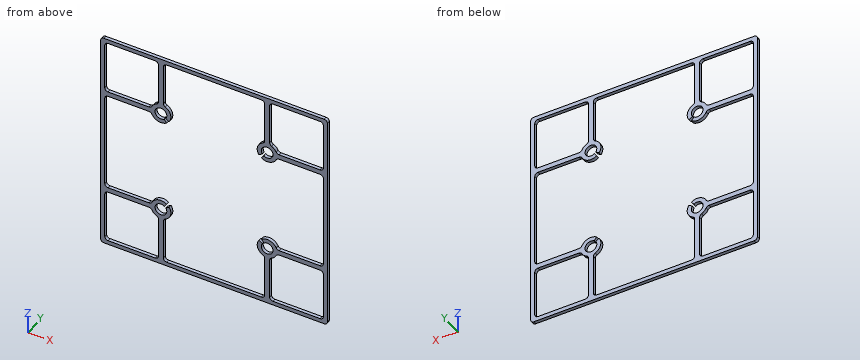
from build123d import *

# Parameters (mm, degrees)
BOSS_EXTRUDE2_DEPTH = 2


with BuildPart() as part:
    # Sketch1 → Boss-Extrude2 (new body)
    with BuildSketch(Plane(origin=(0, 0, 0), x_dir=(1, 0, 0), z_dir=(0, 1, 0))):
        with BuildLine():
            Line((69.363368179, -67.363368179), (69.363368179, 67.363368179))
            ThreePointArc((69.363368179, 67.363368179), (68.777581741, 68.777581741), (67.363368179, 69.363368179))
            Line((67.363368179, 69.363368179), (-67.363368179, 69.363368179))
            ThreePointArc((-67.363368179, 69.363368179), (-68.777581741, 68.777581741), (-69.363368179, 67.363368179))
            Line((-69.363368179, 67.363368179), (-69.363368179, -67.363368179))
            ThreePointArc((-69.363368179, -67.363368179), (-68.777581741, -68.777581741), (-67.363368179, -69.363368179))
            Line((-67.363368179, -69.363368179), (67.363368179, -69.363368179))
            ThreePointArc((67.363368179, -69.363368179), (68.777581741, -68.777581741), (69.363368179, -67.363368179))
        make_face()
        with BuildLine():
            Line((66.863368179, -64.863368179), (66.863368179, -35.99568434))
            ThreePointArc((66.863368179, -35.99568434), (66.277581741, -34.581470778), (64.863368179, -33.99568434))
            Line((64.863368179, -33.99568434), (39.806859174, -33.99568434))
            ThreePointArc((39.806859174, -33.99568434), (38.740619021, -34.303605165), (38.002696415, -35.132552404))
            ThreePointArc((38.002696415, -35.132552404), (36.814625157, -36.812077197), (35.135802469, -38.001140368))
            ThreePointArc((35.135802469, -38.001140368), (34.307605976, -38.739052609), (34, -39.804792947))
            Line((34, -39.804792947), (34, -64.863368179))
            ThreePointArc((34, -64.863368179), (34.585786438, -66.277581741), (36, -66.863368179))
            Line((36, -66.863368179), (64.863368179, -66.863368179))
            ThreePointArc((64.863368179, -66.863368179), (66.277581741, -66.277581741), (66.863368179, -64.863368179))
        make_face(mode=Mode.SUBTRACT)
        with BuildLine():
            Line((-64.863368179, 66.863368179), (-36, 66.863368179))
            ThreePointArc((-36, 66.863368179), (-34.585786438, 66.277581741), (-34, 64.863368179))
            Line((-34, 64.863368179), (-34, 39.804792947))
            ThreePointArc((-34, 39.804792947), (-34.307605976, 38.739052609), (-35.135802469, 38.001140368))
            ThreePointArc((-35.135802469, 38.001140368), (-36.814625157, 36.812077197), (-38.002696415, 35.132552404))
            ThreePointArc((-38.002696415, 35.132552404), (-38.740619021, 34.303605165), (-39.806859174, 33.99568434))
            Line((-39.806859174, 33.99568434), (-64.863368179, 33.99568434))
            ThreePointArc((-64.863368179, 33.99568434), (-66.277581741, 34.581470778), (-66.863368179, 35.99568434))
            Line((-66.863368179, 35.99568434), (-66.863368179, 64.863368179))
            ThreePointArc((-66.863368179, 64.863368179), (-66.277581741, 66.277581741), (-64.863368179, 66.863368179))
        make_face(mode=Mode.SUBTRACT)
        with BuildLine():
            Line((-66.863368179, -64.863368179), (-66.863368179, -35.99568434))
            ThreePointArc((-66.863368179, -35.99568434), (-66.277581741, -34.581470778), (-64.863368179, -33.99568434))
            Line((-64.863368179, -33.99568434), (-39.806859174, -33.99568434))
            ThreePointArc((-39.806859174, -33.99568434), (-38.740619021, -34.303605165), (-38.002696415, -35.132552404))
            ThreePointArc((-38.002696415, -35.132552404), (-36.814625157, -36.812077197), (-35.135802469, -38.001140368))
            ThreePointArc((-35.135802469, -38.001140368), (-34.307605976, -38.739052609), (-34, -39.804792947))
            Line((-34, -39.804792947), (-34, -64.863368179))
            ThreePointArc((-34, -64.863368179), (-34.585786438, -66.277581741), (-36, -66.863368179))
            Line((-36, -66.863368179), (-64.863368179, -66.863368179))
            ThreePointArc((-64.863368179, -66.863368179), (-66.277581741, -66.277581741), (-66.863368179, -64.863368179))
        make_face(mode=Mode.SUBTRACT)
        with BuildLine():
            Line((36, 66.863368179), (64.863368179, 66.863368179))
            ThreePointArc((64.863368179, 66.863368179), (66.277581741, 66.277581741), (66.863368179, 64.863368179))
            Line((66.863368179, 64.863368179), (66.863368179, 35.99568434))
            ThreePointArc((66.863368179, 35.99568434), (66.277581741, 34.581470778), (64.863368179, 33.99568434))
            Line((64.863368179, 33.99568434), (39.806859174, 33.99568434))
            ThreePointArc((39.806859174, 33.99568434), (38.740619021, 34.303605165), (38.002696415, 35.132552404))
            ThreePointArc((38.002696415, 35.132552404), (36.814625157, 36.812077197), (35.135802469, 38.001140368))
            ThreePointArc((35.135802469, 38.001140368), (34.307605976, 38.739052609), (34, 39.804792947))
            Line((34, 39.804792947), (34, 64.863368179))
            ThreePointArc((34, 64.863368179), (34.585786438, 66.277581741), (36, 66.863368179))
        make_face(mode=Mode.SUBTRACT)
        with BuildLine():
            Line((-30.435124829, 29.551052641), (-29.001183738, 27.50317253))
            ThreePointArc((-29.001183738, 27.50317253), (-34.049623523, 26.600112973), (-38.002696415, 29.867447596))
            ThreePointArc((-38.002696415, 29.867447596), (-38.740619021, 30.696394835), (-39.806859174, 31.00431566))
            Line((-39.806859174, 31.00431566), (-64.863368179, 31.00431566))
            ThreePointArc((-64.863368179, 31.00431566), (-66.277581741, 30.418529222), (-66.863368179, 29.00431566))
            Line((-66.863368179, 29.00431566), (-66.863368179, -29.00431566))
            ThreePointArc((-66.863368179, -29.00431566), (-66.277581741, -30.418529222), (-64.863368179, -31.00431566))
            Line((-64.863368179, -31.00431566), (-39.806859174, -31.00431566))
            ThreePointArc((-39.806859174, -31.00431566), (-38.740619021, -30.696394835), (-38.002696415, -29.867447596))
            ThreePointArc((-38.002696415, -29.867447596), (-34.049623523, -26.600112973), (-29.001183738, -27.50317253))
            Line((-29.001183738, -27.50317253), (-30.435124829, -29.551052641))
            ThreePointArc((-30.435124829, -29.551052641), (-35.045584412, -35.045584412), (-29.551052641, -30.435124829))
            Line((-29.551052641, -30.435124829), (-27.50317253, -29.001183738))
            ThreePointArc((-27.50317253, -29.001183738), (-26.599655537, -34.04788088), (-29.864197531, -38.001140368))
            ThreePointArc((-29.864197531, -38.001140368), (-30.692394024, -38.739052609), (-31, -39.804792947))
            Line((-31, -39.804792947), (-31, -64.863368179))
            ThreePointArc((-31, -64.863368179), (-30.414213562, -66.277581741), (-29, -66.863368179))
            Line((-29, -66.863368179), (29, -66.863368179))
            ThreePointArc((29, -66.863368179), (30.414213562, -66.277581741), (31, -64.863368179))
            Line((31, -64.863368179), (31, -39.804792947))
            ThreePointArc((31, -39.804792947), (30.692394024, -38.739052609), (29.864197531, -38.001140368))
            ThreePointArc((29.864197531, -38.001140368), (26.599655537, -34.04788088), (27.50317253, -29.001183738))
            Line((27.50317253, -29.001183738), (29.551052641, -30.435124829))
            ThreePointArc((29.551052641, -30.435124829), (35.045584412, -35.045584412), (30.435124829, -29.551052641))
            Line((30.435124829, -29.551052641), (29.001183738, -27.50317253))
            ThreePointArc((29.001183738, -27.50317253), (34.049623523, -26.600112973), (38.002696415, -29.867447596))
            ThreePointArc((38.002696415, -29.867447596), (38.740619021, -30.696394835), (39.806859174, -31.00431566))
            Line((39.806859174, -31.00431566), (64.863368179, -31.00431566))
            ThreePointArc((64.863368179, -31.00431566), (66.277581741, -30.418529222), (66.863368179, -29.00431566))
            Line((66.863368179, -29.00431566), (66.863368179, 29.00431566))
            ThreePointArc((66.863368179, 29.00431566), (66.277581741, 30.418529222), (64.863368179, 31.00431566))
            Line((64.863368179, 31.00431566), (39.806859174, 31.00431566))
            ThreePointArc((39.806859174, 31.00431566), (38.740619021, 30.696394835), (38.002696415, 29.867447596))
            ThreePointArc((38.002696415, 29.867447596), (34.049623523, 26.600112973), (29.001183738, 27.50317253))
            Line((29.001183738, 27.50317253), (30.435124829, 29.551052641))
            ThreePointArc((30.435124829, 29.551052641), (35.045584412, 35.045584412), (29.551052641, 30.435124829))
            Line((29.551052641, 30.435124829), (27.50317253, 29.001183738))
            ThreePointArc((27.50317253, 29.001183738), (26.599655537, 34.04788088), (29.864197531, 38.001140368))
            ThreePointArc((29.864197531, 38.001140368), (30.692394024, 38.739052609), (31, 39.804792947))
            Line((31, 39.804792947), (31, 64.863368179))
            ThreePointArc((31, 64.863368179), (30.414213562, 66.277581741), (29, 66.863368179))
            Line((29, 66.863368179), (-29, 66.863368179))
            ThreePointArc((-29, 66.863368179), (-30.414213562, 66.277581741), (-31, 64.863368179))
            Line((-31, 64.863368179), (-31, 39.804792947))
            ThreePointArc((-31, 39.804792947), (-30.692394024, 38.739052609), (-29.864197531, 38.001140368))
            ThreePointArc((-29.864197531, 38.001140368), (-26.599655537, 34.04788088), (-27.50317253, 29.001183738))
            Line((-27.50317253, 29.001183738), (-29.551052641, 30.435124829))
            ThreePointArc((-29.551052641, 30.435124829), (-35.045584412, 35.045584412), (-30.435124829, 29.551052641))
        make_face(mode=Mode.SUBTRACT)
    extrude(amount=BOSS_EXTRUDE2_DEPTH)


solid = part.part
Design review of the part built by this model. Coordinates are the model's own, in mm. Coordinates: 2 decimals unless noted, no trailing zeros. Loops run counter-clockwise (first coordinate to the right, second up) from the corner with the lowest first, then second, coordinate; pieces in that order, holes last. Notation, with made-up numbers: (22.25, 45.25) -> (68.25, 45.25) arc R16 ccw to (68.25, 64.25) -> close; hole circle Ø4 at (79, 9). An arc over 180 degrees is marked (long way). Use a Markdown table: item, result. Add a question column.
Item 1: We need section D-D, the plane y = 1.7. Count the separate pieces of the cut face and the enclosed holes in it, and give its area (3 significant figures).
Item 2: We need section C-C, the plane z = 2. Write out the cut boundary in (x, y), and give its area (3 significant figures).
Item 3: We need section B-B, the plane x = 50.5. Write out the cut boundary in (y, z), and give its area (3 significant figures).
Item 4: Wall thickness on L1, parallel to Z at x = -39.5, y = 1.55; L2, parallel to Z at x = 32.5, y = 0.95; L3, parallel to X at y = 1.55, z = 49.5: over which ranges is each line inside the solid? List them lowest first. Write a range as from..to.
Item 5: Clearance check with a flat-ended pin moving along its axis: P1, Ø6.5, axis at x = 32.5, z = 32.5, coming from the -Y side. State where the tip first meets the part, or that it passes through.
Item 6: We need section A-A, the plane z = 56.5. Write out the cut boundary in (x, y).
Numbers:
| question | item | result |
|---|---|---|
| 1 | separate pieces | 1 |
| 1 | enclosed holes | 5 |
| 1 | area | 2,350 mm^2 |
| 2 | outline | (-69.36, 0) -> (-66.86, 0) -> (-66.86, 2) -> (-69.36, 2) -> close; (66.86, 0) -> (69.36, 0) -> (69.36, 2) -> (66.86, 2) -> close |
| 2 | area | 10.0 mm^2 |
| 3 | outline | (0, -69.36) -> (2, -69.36) -> (2, -66.86) -> (0, -66.86) -> close; (0, -34) -> (2, -34) -> (2, -31) -> (0, -31) -> close; (0, 31) -> (2, 31) -> (2, 34) -> (0, 34) -> close; (0, 66.86) -> (2, 66.86) -> (2, 69.36) -> (0, 69.36) -> close |
| 3 | area | 22.0 mm^2 |
| 4 | L1 | z = -69.36..-66.86, -34.02..-30.98, 30.98..34.02, 66.86..69.36 |
| 4 | L2 | z = -69.36..-36.1, -28.9..-26.4, 26.4..28.9, 36.1..69.36 |
| 4 | L3 | x = -69.36..-66.86, -34..-31, 31..34, 66.86..69.36 |
| 5 | P1 | passes through |
| 6 | outline | (-69.36, 0) -> (-66.86, 0) -> (-66.86, 2) -> (-69.36, 2) -> close; (-34, 0) -> (-31, 0) -> (-31, 2) -> (-34, 2) -> close; (31, 0) -> (34, 0) -> (34, 2) -> (31, 2) -> close; (66.86, 0) -> (69.36, 0) -> (69.36, 2) -> (66.86, 2) -> close |
